Design review of the part built by this model. Coordinates are the model's own, in mm. A direction names the side the tool comes from. Round coordinates to 2 decimals unless told otherwise and drop trailing zeros. Order: outer loops, then holes, each group sorted by start corner. A loop starts at its lowest first (then second) coordinate and runs counter-clockwise, first axis right, second up. Notation, with made-up numbers: (-24, -18) - (-12, -18) arc R18 ccw to (-12, -13) - close; hole circle Ø11 at (-2, 48.5). An arc over 180 degrees is marked (long way). Use CSV: the item, a comma, the result in double quotes. Start each with the question number.
from build123d import *

# Parameters (mm, degrees)
SKETCH1_R               = 400
BOSS_EXTRUDE1_DEPTH     = 10
BOSS_EXTRUDE5_DEPTH     = 130
BOSS_EXTRUDE6_START     = -30
SKETCH1_4_R             = 400
BOSS_EXTRUDE6_DEPTH     = 30
SKETCH4_W               = 17
SKETCH4_H               = 369.202632894
SKETCH4_H_2             = 374.689720856
BOSS_EXTRUDE7_DEPTH     = 450
CUT_EXTRUDE1_DEPTH      = 789.823332566
CUT_EXTRUDE1_DEPTH_BACK = 300
SKETCH6_R               = 13.5
CUT_EXTRUDE2_DEPTH      = 300


with BuildPart() as part:
    # Sketch1 → Boss-Extrude1 (new body)
    with BuildSketch(Plane(origin=(0, 0, 0), x_dir=(1, 0, 0), z_dir=(0, 1, 0))):
        with Locations(Location((0, 0, 0), (0, 0, 270))):
            Circle(SKETCH1_R)
    extrude(amount=BOSS_EXTRUDE1_DEPTH)

    # Sketch3 → Boss-Extrude5 (add)
    with BuildSketch(Plane(origin=(0, 10, 0), x_dir=(1, 0, 0), z_dir=(0, 1, 0))):
        with BuildLine():
            Line((-4.6, -30.015), (4.6, -30.015))
            Line((4.6, -30.015), (4.6, -24.573156085))
            ThreePointArc((4.6, -24.573156085), (0, 25), (-4.6, -24.573156085))
            Line((-4.6, -24.573156085), (-4.6, -30.015))
        make_face()
    extrude(amount=BOSS_EXTRUDE5_DEPTH)

    # Sketch1_4 → Boss-Extrude6 (add)
    with BuildSketch(Plane(origin=(0, 0, 0), x_dir=(1, 0, 0), z_dir=(0, 1, 0)).offset(BOSS_EXTRUDE6_START)):
        with Locations(Location((0, 0, 0), (0, 0, 270))):
            Circle(SKETCH1_4_R)
    extrude(amount=BOSS_EXTRUDE6_DEPTH)

    # Sketch4 → Boss-Extrude7 (add)
    with BuildSketch(Plane.XZ.offset(30)):
        with Locations((-73, -0.045418377)):
            Rectangle(SKETCH4_W, SKETCH4_H)
        with Locations((73, -2.788962358)):
            Rectangle(SKETCH4_W, SKETCH4_H_2)
    extrude(amount=BOSS_EXTRUDE7_DEPTH)

    # Sketch5 → Cut-Extrude1 (cut, two sides: drawn at the far end of the back side and taken through both)
    with BuildSketch(Plane(origin=(81.5, 0, 0), x_dir=(0, 0, -1), z_dir=(1, 0, 0)).offset(-CUT_EXTRUDE1_DEPTH_BACK)):
        Polygon((-184.55589807, -287.770569758), (-72.211037642, -480), (-184.55589807, -480), align=None)
        Polygon((77.788962358, -480), (190.133822786, -287.770569758), (190.133822786, -480), align=None)
    extrude(amount=CUT_EXTRUDE1_DEPTH + CUT_EXTRUDE1_DEPTH_BACK, mode=Mode.SUBTRACT)

    # Sketch6 → Cut-Extrude2 (cut)
    with BuildSketch(Plane.ZY.offset(81.5)):
        with Locations((0, -410)):
            Circle(SKETCH6_R)
    extrude(amount=-CUT_EXTRUDE2_DEPTH, mode=Mode.SUBTRACT)


solid = part.part
Q1. Clearance check with flat-ended pins moving along their axes: pin 1 (16 mm diameter, centred on y = -410, z = 0, fed in from +X); pin 2 (1.6 mm diameter, centred on y = 64.5, z = 27, fed in from -X); pin 3 (18.5 mm diameter, centred on x = 76.5, y = -155, fed in from +Z); pin 4 (8 mm diameter, centred on x = 87, z = -305.5, fed in from -Y). State where each tip first meets the part, or that it passes through.
Q2. Take a section at D-D (z = -100). State the section outline as (x, y) points.
Q3. Take a section at A-A (z = 0). State the section outline as (x, y) points.
Q4. For L1, parallel to X at y = -338, z = 104; L2, parallel to Y at x = 72, z = 0; L3, parallel to Y at x = -63, z = -291, list the stretches that pass through material, from the lowest coordinate up. Write a range as [from, to].
Q5. Tool access review of faces 1 (the flat face through (72.881, -385.231, -133.175)), 2 (the flat face through (-81.5, -252, -3)), 3 (the cylindrical face through (120.15, -10.28, 381.53)), 4 (the flat face through (81.5, -252, -5)), 5 (the flat face through (-64.5, -252, -3)): name each direction out of +Z, -Z, +X, -X, +Y, -Y from which nothing blocks a thin tool from reaching the whole face with its end or side.
Q6. Take a section at C-C (y = -410). State the section outline as (x, z) points.
Q7. The part is to be moulded in two halves that separate along Y. For faces 6 (the cylindrical face through (72.881, -396.615, -1.757)), 7 (the flat face through (-73.12, -389.86, -130.47)), 8 (the cylindrical face through (1.03, 74.09, -24.98)), 9 (the flat face through (0, 140, 2)), say which applies: +Y half, -Y half, draft (parallel to the pull), parting line (faces both ways), or undercut.
Q8. Take a section at B-B (y = -181). State the section outline as (x, z) points, plus the area to 3 significant figures.
Findings below:
1,pin 1,"passes through"
1,pin 2,"stops at x = -4.6"
1,pin 3,"stops at z = 184.56"
1,pin 4,"stops at y = -30"
2,outline,"(-387.3, -30) - (-81.5, -30) - (-81.5, -442) - (-64.5, -442) - (-64.5, -30) - (64.5, -30) - (64.5, -442) - (81.5, -442) - (81.5, -30) - (387.3, -30) - (387.3, 10) - (-387.3, 10) - close"
3,outline,"(-400, -30) - (-81.5, -30) - (-81.5, -396.5) - (-64.5, -396.5) - (-64.5, -30) - (64.5, -30) - (64.5, -396.5) - (81.5, -396.5) - (81.5, -30) - (400, -30) - (400, 10) - (25, 10) - (25, 140) - (-25, 140) - (-25, 10) - (-400, 10) - close; (-81.5, -480) - (-64.5, -480) - (-64.5, -423.5) - (-81.5, -423.5) - close; (64.5, -480) - (81.5, -480) - (81.5, -423.5) - (64.5, -423.5) - close"
4,L1,"x = [-81.5, -64.5], [64.5, 81.5]"
4,L2,"y = [-480, -423.5], [-396.5, 10]"
4,L3,"y = [-30, 10]"
5,face 1,"-Z, +X, -X, -Y"
5,face 2,"+Z, -Z, -X, -Y"
5,face 3,"+Y, -Y"
5,face 4,"+Z, -Z, +X, -Y"
5,face 5,"+Z, -Z, -Y"
6,outline,"(-81.5, -118.7) - (-64.5, -118.7) - (-64.5, -13.5) - (-81.5, -13.5) - close; (-81.5, 13.5) - (-64.5, 13.5) - (-64.5, 113.12) - (-81.5, 113.12) - close; (64.5, -118.7) - (81.5, -118.7) - (81.5, -13.5) - (64.5, -13.5) - close; (64.5, 13.5) - (81.5, 13.5) - (81.5, 113.12) - (64.5, 113.12) - close"
7,face 6,"undercut"
7,face 7,"-Y half"
7,face 8,"draft"
7,face 9,"+Y half"
8,outline,"(-81.5, -184.65) - (-64.5, -184.65) - (-64.5, 184.56) - (-81.5, 184.56) - close; (64.5, -190.13) - (81.5, -190.13) - (81.5, 184.56) - (64.5, 184.56) - close"
8,area,"12,600 mm^2"
